```python
from build123d import *

# Parameters (mm, degrees)
SKETCH1_W                                      = 19.98
SKETCH1_H                                      = 128.4
BOSS_EXTRUDE1_DEPTH                            = 2.5
CUT_EXTRUDE1_DEPTH                             = 127.049239982
CUT_EXTRUDE2_DEPTH                             = 127.049239982
SKETCH4_W                                      = 3.9
SKETCH4_H                                      = 14.6
CUT_EXTRUDE3_DEPTH                             = 127.049239982
F_3_0_3_DIAMETER_HOLE1_D                       = 3
CSK_FOR_M2_5_FLAT_HEAD_MACHINE_SCREW1_AT_COUNT = 2
CSK_FOR_M2_5_FLAT_HEAD_MACHINE_SCREW1_AT_PITCH = 99.130249672
USB_DEPTH                                      = 127.049239982
SKETCH10_R                                     = 1.3
LEDS_DEPTH                                     = 127.049239982
SKETCH11_R                                     = 2.5
RESET_SWITCH_DEPTH                             = 127.049239982
SKETCH13_W                                     = 9
SKETCH13_H                                     = 5.5
DISABLE_COMMS_DEPTH                            = 127.049239982
SKETCH14_W                                     = 13.2
SKETCH14_H                                     = 17
RJ45_DEPTH                                     = 127.049239982
SKETCH15_W                                     = 10.8
SKETCH15_H                                     = 18
OUTPUT_DEPTH                                   = 127.049239982
SKETCH16_W                                     = 11.5
SKETCH16_H                                     = 10
POWER_DEPTH                                    = 127.049239982
FILLETS_R                                      = 0.5


with BuildPart() as part:
    # Sketch1 → Boss-Extrude1 (new body)
    with BuildSketch(Plane.XY.offset(2.5)):
        with Locations((2.54, 61.2)):
            Rectangle(SKETCH1_W, SKETCH1_H)
    extrude(amount=-BOSS_EXTRUDE1_DEPTH)

    # Sketch2 → Cut-Extrude1 (cut, through all)
    with BuildSketch(Plane.XY.offset(2.5)):
        with BuildLine():
            Line((2.445403852, 124.05), (-2.445403852, 124.05))
            ThreePointArc((-2.445403852, 124.05), (-2.95, 122.4), (-2.445403852, 120.75))
            Line((-2.445403852, 120.75), (2.445403852, 120.75))
            ThreePointArc((2.445403852, 120.75), (2.95, 122.4), (2.445403852, 124.05))
        make_face()
    extrude(amount=-CUT_EXTRUDE1_DEPTH, mode=Mode.SUBTRACT)

    # Sketch3 → Cut-Extrude2 (cut, through all)
    with BuildSketch(Plane.XY.offset(2.5)):
        with BuildLine():
            Line((7.525403852, 1.65), (2.634596148, 1.65))
            ThreePointArc((2.634596148, 1.65), (2.13, 0), (2.634596148, -1.65))
            Line((2.634596148, -1.65), (7.525403852, -1.65))
            ThreePointArc((7.525403852, -1.65), (8.03, 0), (7.525403852, 1.65))
        make_face()
    extrude(amount=-CUT_EXTRUDE2_DEPTH, mode=Mode.SUBTRACT)

    # Sketch4 → Cut-Extrude3 (cut, through all)
    with BuildSketch(Plane(origin=(0, 0, 0), x_dir=(-1, 0, 0), z_dir=(0, 0, -1))):
        with Locations((1.87, 8.5)):
            Rectangle(SKETCH4_W, SKETCH4_H)
    extrude(amount=-CUT_EXTRUDE3_DEPTH, mode=Mode.SUBTRACT)

    # Ø3.0 (3) Diameter Hole1 (through all)
    with Locations(Plane.XY.offset(2.5)):
        with Locations((-3.95, 119.1)):
            Hole(F_3_0_3_DIAMETER_HOLE1_D / 2)

    # Sketch7 → CSK for M2.5 Flat Head Machine Screw1 (revolve, cut)
    with BuildSketch(Plane(origin=(5.08, 11.7, 2.5), x_dir=(0, -1, 0), z_dir=(1, 0, 0))):
        Polygon((0, 0), (0, 2.5), (1.35, 2.5), (1.35, 1.5), (2.5, 0.35), (2.5, 0), align=None)
    csk_for_m2_5_flat_head_machine_screw1 = revolve(axis=Axis((5.08, 11.7, 8.85), (0, 0, -1)), mode=Mode.SUBTRACT)

    # CSK for M2.5 Flat Head Machine Screw1 at: CSK for M2.5 Flat Head Machine Screw1 ×2
    with Locations(*[Vector(-0.05124570972853528, 0.9986860754183062, 0) * (i * CSK_FOR_M2_5_FLAT_HEAD_MACHINE_SCREW1_AT_PITCH) for i in range(1, CSK_FOR_M2_5_FLAT_HEAD_MACHINE_SCREW1_AT_COUNT)]):
        add(csk_for_m2_5_flat_head_machine_screw1, mode=Mode.SUBTRACT)

    # Sketch9 → USB (cut, through all)
    with BuildSketch(Plane.XY.offset(2.5)):
        Polygon((-3.82, 19.95), (1.78, 19.95), (1.78, 32.45), (-3.82, 32.45), (-6.95, 32.45), (-6.95, 19.95), align=None)
    extrude(amount=-USB_DEPTH, mode=Mode.SUBTRACT)

    # Sketch10 → LEDs (cut, through all)
    with BuildSketch(Plane.XY.offset(2.5)):
        with Locations((-1.28, 34.65)):
            Circle(SKETCH10_R)
        with Locations((3.8, 34.65)):
            Circle(SKETCH10_R)
    extrude(amount=-LEDS_DEPTH, mode=Mode.SUBTRACT)

    # Sketch11 → Reset switch (cut, through all)
    with BuildSketch(Plane.XY.offset(2.5)):
        with Locations((-1.32, 42.7)):
            Circle(SKETCH11_R)
    extrude(amount=-RESET_SWITCH_DEPTH, mode=Mode.SUBTRACT)

    # Sketch13 → Disable comms (cut, through all)
    with BuildSketch(Plane.XY.offset(2.5)):
        with Locations((0.505, 51.2)):
            Rectangle(SKETCH13_W, SKETCH13_H)
    extrude(amount=-DISABLE_COMMS_DEPTH, mode=Mode.SUBTRACT)

    # Sketch14 → RJ45 (cut, through all)
    with BuildSketch(Plane.XY.offset(2.5)):
        with Locations((2.78, 63.2)):
            Rectangle(SKETCH14_W, SKETCH14_H)
    extrude(amount=-RJ45_DEPTH, mode=Mode.SUBTRACT)

    # Sketch15 → Output (cut, through all)
    with BuildSketch(Plane.XY.offset(2.5)):
        with Locations((1.58, 81.2)):
            Rectangle(SKETCH15_W, SKETCH15_H)
    extrude(amount=-OUTPUT_DEPTH, mode=Mode.SUBTRACT)

    # Sketch16 → Power (cut, through all)
    with BuildSketch(Plane.XY.offset(2.5)):
        with Locations((1.93, 96.2)):
            Rectangle(SKETCH16_W, SKETCH16_H)
    extrude(amount=-POWER_DEPTH, mode=Mode.SUBTRACT)

    # Fillets
    fillets_edges = [part.edges().sort_by_distance(p)[0] for p in [
        (5.005, 53.95, 1.25),
        (5.005, 48.45, 1.25),
        (-3.995, 48.45, 1.25),
        (-3.995, 53.95, 1.25),
        (9.38, 54.7, 1.25),
        (-3.82, 54.7, 1.25),
        (-3.82, 71.7, 1.25),
        (9.38, 71.7, 1.25),
        (6.98, 72.2, 1.25),
        (-3.82, 72.2, 1.25),
        (-3.82, 90.2, 1.25),
        (6.98, 90.2, 1.25),
        (7.68, 91.2, 1.25),
        (-3.82, 91.2, 1.25),
        (-3.82, 101.2, 1.25),
        (7.68, 101.2, 1.25),
        (-3.82, 15.8, 1.25),
        (-3.82, 1.2, 1.25),
        (0.08, 1.2, 1.25),
        (0.08, 15.8, 1.25),
        (-6.95, 19.95, 1.25),
        (-6.95, 32.45, 1.25),
        (1.78, 32.45, 1.25),
        (1.78, 19.95, 1.25),
    ]]
    fillet(fillets_edges, radius=FILLETS_R)


solid = part.part
```
The model under review builds one solid part; all positions refer to its coordinate system, in mm. Round coordinates to 2 decimals unless told otherwise and drop trailing zeros. Order: outer loops, then holes, each group sorted by start corner. A loop starts at its lowest first (then second) coordinate and runs counter-clockwise, first axis right, second up. Notation, with made-up numbers: (31.5, 61.25) -> (62.5, 61.25) arc R24 cw to (62.5, 92.25) -> close; hole circle Ø11 at (4, 18). An arc over 180 degrees is marked (long way). One line per item, written item: value. Start each with the question number.
Q1. Clearance check with flat-ended pins moving along their axes: pin 1 Ø4.5 at (x, y) = (0, 110.7) entering from +Z; pin 2 Ø2 at (x, y) = (-4, 23.5) entering from -Z; pin 3 Ø4 at (x, y) = (3.5, 99.5) entering from +Z. State where each tip first meets the part, or that it passes through.
Q2. Wall thickness on line 1 (X direction, y = 11.7, z = 2.3); line 2 (X direction, y = 11.7, z = 0.5); line 3 (X direction, y = 119.1, z = 2): over which ranges is each line inside the solid? List them lowest first.
Q3. Take a section at A-A (y = 98). Write out the cut boundary in (x, z).
Q4. Mouldability with a two-part tool opening along X and no side actions: class faces 1 (the face through (12.53, 60, 1)), 2 (the face through (2, 72.2, 1)), 3 (the face through (-4, 62, 2.5)) as released by +X, released by -X, zero draft, split by the parting line, or undercut.
Q5. Take a section at B-B (y = 119.1). Write out the cut boundary in (x, z), and give its area (4 significant figures).
Q6. Take a section at C-C (z = 1.5). Count the separate pieces of the cut face and the enclosed holes in it, and give its area (3 significant figures).
Reported:
1. pin 1: stops at z = 1.9
1. pin 2: passes through
1. pin 3: stops at z = 2.5
2. line 1: x = -7.45 to -3.82, 0.08 to 2.58, 7.58 to 12.53
2. line 2: x = -7.45 to -3.82, 0.08 to 3.73, 6.43 to 12.53
2. line 3: x = -7.45 to -5.45, -2.45 to 12.53
3. outline: (-7.45, 0) -> (-3.82, 0) -> (-3.82, 2.5) -> (-7.45, 2.5) -> close; (7.68, 0) -> (12.53, 0) -> (12.53, 2.5) -> (7.68, 2.5) -> close
4. face 1: released by +X
4. face 2: undercut
4. face 3: zero draft
5. outline: (-7.45, 0) -> (-5.45, 0) -> (-5.45, 2.5) -> (-7.45, 2.5) -> close; (-2.45, 0) -> (12.53, 0) -> (12.53, 2.5) -> (-2.45, 2.5) -> close
5. area: 42.45 mm2
6. separate pieces: 1
6. enclosed holes: 14
6. area: 1,720 mm2
